Verification items for the finished model (mm, model axes). A direction names the side the tool comes from. Coordinates: 2 decimals unless noted, no trailing zeros. Order: outer loops, then holes, each group sorted by start corner. A loop starts at its lowest first (then second) coordinate and runs counter-clockwise, first axis right, second up. Notation, with made-up numbers: M 23,62.5 L 82,62.5 A15 cw 82,87.5 Z; hole C 74,-2.75 d10. An arc over 180 degrees is marked long. Answer as a JSON object with one key per item and string values. Group by question number.
(1) Cross-section at A-A (y = 12). Enter the section's corners in (x, z).
(2) Material ranges on line 1 (X direction, y = 4, z = 0.8); line 2 (X direction, y = 57, z = 1.85); line 3 (X direction, y = 35, z = 1.65), recorded low to high.
(3) Gauge pin test, flat ends, axial feed: pin 1 Ø1.3 at (y, z) = (37, 2) entering from +X; pin 2 Ø1.5 at (x, z) = (17, 4) entering from +Y; pin 3 Ø2 at (x, z) = (38.5, 1.5) entering from -Y. Record the tip position at first contact, or that the pin passes through.
(4) Mould release check, pull along Y, two halves, no side actions. Record for faces 5 (the face through (58, 22.2, 2)), 6 (the face through (0, 54, 2)), 7 (the face through (55.5, 39, 2)): released by +Y, released by -Y, zero draft, split by the parting line, or undercut.
(5) Access from +Z, -Z, +X, -X, +Y, -Y to the whole of each face (thin tool, end or side, straight path). Record for faces 1 (the face through (15.6, 58, 2)), 2 (the face through (55.5, 17, 2)), 3 (the face through (2, 48.9, 2)), 4 (the face through (33.3, 2, 2)).
(6) Cross-section at B-B (x = 17). Enter the section's corners in (y, z), plus the area to 4 significant figures.
from build123d import *

# Parameters (mm, degrees)
SKETCH1_W           = 60
SKETCH1_H           = 60
BOSS_EXTRUDE1_DEPTH = 4.5
CAVITY1_OUTLINE_W   = 11.1
CAVITY1_OUTLINE_H   = 4.5
CAVITY1_DEPTH       = 4.5
CAVITY1_START       = 55.5
CAVITY1_2_OUTLINE_W = 11.1
CAVITY1_2_OUTLINE_H = 4.5
CAVITY1_2_DEPTH     = 4.5
CAVITY1_START_2     = 15.6
CAVITY1_3_OUTLINE_W = 4.5
CAVITY1_3_OUTLINE_H = 4.5
CAVITY1_3_DEPTH     = 6.6
CAVITY1_START_3     = 37.8
CAVITY1_4_OUTLINE_W = 4.5
CAVITY1_4_OUTLINE_H = 4.5
CAVITY1_4_DEPTH     = 6.6
CAVITY1_START_4     = 11.1
CAVITY1_5_OUTLINE_W = 4.5
CAVITY1_5_OUTLINE_H = 4.5
CAVITY1_5_DEPTH     = 4.5
CAVITY1_START_5     = 22.2
CAVITY1_6_OUTLINE_W = 4.5
CAVITY1_6_OUTLINE_H = 4.5
CAVITY1_6_DEPTH     = 4.5
CAVITY1_START_6     = 33.3
CAVITY1_7_OUTLINE_W = 4.5
CAVITY1_7_OUTLINE_H = 4.5
CAVITY1_7_DEPTH     = 4.5
CAVITY1_START_7     = 44.4
CAVITY1_8_OUTLINE_W = 4.5
CAVITY1_8_OUTLINE_H = 4.5
CAVITY1_8_DEPTH     = 4.5


# Read off the part's stored shape, not the designer's step: Cavity1
with BuildPart() as part:
    # Sketch1 → Boss-Extrude1 (new body)
    with BuildSketch(Plane.XY):
        with Locations((30, 30)):
            Rectangle(SKETCH1_W, SKETCH1_H)
    extrude(amount=BOSS_EXTRUDE1_DEPTH)

    # Cavity1 outline → Cavity1 (cut)
    with BuildSketch(Plane.YZ):
        with Locations((21.15, 2.25)):
            Rectangle(CAVITY1_OUTLINE_W, CAVITY1_OUTLINE_H)
        with Locations((43.35, 2.25)):
            Rectangle(CAVITY1_OUTLINE_W, CAVITY1_OUTLINE_H)
    extrude(amount=CAVITY1_DEPTH, mode=Mode.SUBTRACT)

    # Cavity1 2 outline → Cavity1 2 (cut)
    with BuildSketch(Plane.YZ.offset(CAVITY1_START)):
        with Locations((16.65, 2.25)):
            Rectangle(CAVITY1_2_OUTLINE_W, CAVITY1_2_OUTLINE_H)
        with Locations((38.85, 2.25)):
            Rectangle(CAVITY1_2_OUTLINE_W, CAVITY1_2_OUTLINE_H)
    extrude(amount=CAVITY1_2_DEPTH, mode=Mode.SUBTRACT)

    # Cavity1 3 outline → Cavity1 3 (cut)
    with BuildSketch(Plane.YZ.offset(CAVITY1_START_2)):
        with Locations((2.25, 2.25)):
            Rectangle(CAVITY1_3_OUTLINE_W, CAVITY1_3_OUTLINE_H)
        with Locations((57.75, 2.25)):
            Rectangle(CAVITY1_3_OUTLINE_W, CAVITY1_3_OUTLINE_H)
    extrude(amount=CAVITY1_3_DEPTH, mode=Mode.SUBTRACT)

    # Cavity1 4 outline → Cavity1 4 (cut)
    with BuildSketch(Plane.YZ.offset(CAVITY1_START_3)):
        with Locations((2.25, 2.25)):
            Rectangle(CAVITY1_4_OUTLINE_W, CAVITY1_4_OUTLINE_H)
        with Locations((57.75, 2.25)):
            Rectangle(CAVITY1_4_OUTLINE_W, CAVITY1_4_OUTLINE_H)
    extrude(amount=CAVITY1_4_DEPTH, mode=Mode.SUBTRACT)

    # Cavity1 5 outline → Cavity1 5 (cut)
    with BuildSketch(Plane.YZ.offset(CAVITY1_START_4)):
        with Locations((2.25, 2.25)):
            Rectangle(CAVITY1_5_OUTLINE_W, CAVITY1_5_OUTLINE_H)
    extrude(amount=CAVITY1_5_DEPTH, mode=Mode.SUBTRACT)

    # Cavity1 6 outline → Cavity1 6 (cut)
    with BuildSketch(Plane.YZ.offset(CAVITY1_START_5)):
        with Locations((57.75, 2.25)):
            Rectangle(CAVITY1_6_OUTLINE_W, CAVITY1_6_OUTLINE_H)
    extrude(amount=CAVITY1_6_DEPTH, mode=Mode.SUBTRACT)

    # Cavity1 7 outline → Cavity1 7 (cut)
    with BuildSketch(Plane.YZ.offset(CAVITY1_START_6)):
        with Locations((2.25, 2.25)):
            Rectangle(CAVITY1_7_OUTLINE_W, CAVITY1_7_OUTLINE_H)
    extrude(amount=CAVITY1_7_DEPTH, mode=Mode.SUBTRACT)

    # Cavity1 8 outline → Cavity1 8 (cut)
    with BuildSketch(Plane.YZ.offset(CAVITY1_START_7)):
        with Locations((57.75, 2.25)):
            Rectangle(CAVITY1_8_OUTLINE_W, CAVITY1_8_OUTLINE_H)
    extrude(amount=CAVITY1_8_DEPTH, mode=Mode.SUBTRACT)


solid = part.part
Taken from the geometry:
{
 "1": {"outline": "M 0,0 L 55.5,0 L 55.5,4.5 L 0,4.5 Z"},
 "2": {"line 1": "x = 0 to 11.1, 22.2 to 33.3, 44.4 to 60", "line 2": "x = 0 to 15.6, 26.7 to 37.8, 48.9 to 60", "line 3": "x = 0 to 55.5"},
 "3": {"pin 1": "stops at x = 55.5", "pin 2": "stops at y = 55.5", "pin 3": "stops at y = 4.5"},
 "4": {"face 5": "undercut", "face 6": "zero draft", "face 7": "undercut"},
 "5": {"face 1": "+Z, -Z, +Y", "face 2": "+Z, -Z, +X", "face 3": "+Z, -Z, -X", "face 4": "+Z, -Z, -Y"},
 "6": {"outline": "M 4.5,0 L 55.5,0 L 55.5,4.5 L 4.5,4.5 Z", "area": "229.5 mm²"}
}
